Autodesk Inventor part; units mm, degrees
ref_plane "YZ Plane" through (0, 0, 0) normal (1, 0, 0) x (0, 1, 0)
ref_plane "XZ Plane" through (0, 0, 0) normal (0, 1, 0) x (-1, 0, 0)
ref_plane "XY Plane" through (0, 0, 0) normal (0, 0, 1) x (1, 0, 0)
sketch "Esquisse1" plane through (0, 0, 0) normal (0, 0, 1) x (1, 0, 0)
  line L0 (0, 0) -> (33.8, 0)
  line L1 (0, 0) -> (0, 9.5191)
  line L2 (2.3899, 12.4564) -> (30.1899, 18.2302)
  line L3 (33.8, 15.2929) -> (33.8, 0)
  arc A0 (2.3899, 12.4564) -> (0, 9.5191) centre (3, 9.5191) ccw
  arc A1 (33.8, 15.2929) -> (30.1899, 18.2302) centre (30.8, 15.2929) ccw
  point P0 (0, 11.96)
  point P1 (33.8, 18.98)
  dimension "d0" = 33.8
  dimension "d1" = 18.98
  dimension "d2" = 11.96
  dimension "d3" = 3
  dimension "d4" = 3
extrude "Extrusion1" add sketch "Esquisse1" against normal blind 2
sketch "Esquisse2" plane through (0, 0, 0) normal (0, -1, 0) x (1, 0, 0)
  line L0 (33.8, -2) -> (0, -2)
  line L1 (33.8, -2) -> (0, -2)
  line L2 (0, -2) -> (0, -11)
  line L3 (0, -11) -> (33.8, -11)
  line L4 (33.8, -11) -> (33.8, -2)
  point P0 (33.8, 0)
  dimension "d8" = 9
extrude "Extrusion2" add sketch "Esquisse2" against normal blind 2
sketch "Esquisse3" plane through (33.8, 0, -11) normal (0, 0, -1) x (-1, 0, 0)
  line L0 (0, 2) -> (33.8, 2)
  line L1 (33.8, 2) -> (33.8, 9.5191)
  line L2 (0, 15.2929) -> (0, 2)
  line L3 (0, 15.2929) -> (0, 2)
  line L4 (0, 2) -> (33.8, 2)
  line L5 (3.6101, 18.2302) -> (31.4101, 12.4564)
  arc A0 (3.6101, 18.2302) -> (0, 15.2929) centre (3, 15.2929) ccw
  arc A1 (33.8, 9.5191) -> (31.4101, 12.4564) centre (30.8, 9.5191) ccw
  point P0 (33.8, 0)
  point P1 (33.8, 11.96)
  point P2 (0, 18.98)
  dimension "d11" = 9.96
  dimension "d12" = 16.98
  dimension "d13" = 3
extrude "Extrusion3" add sketch "Esquisse3" against normal blind 2
sketch "Esquisse4" plane through (0, 0, 0) normal (0, 0, 1) x (1, 0, 0)
  line L0 (0, 0) -> (3.39, 0) construction
  line L1 (0, 0) -> (33.8, 0) construction
  line L2 (3.39, 9.1) -> (3.39, 0) construction
  circle A0 centre (3.39, 9.1) radius 2
  circle A1 centre (30.41, 9.1) radius 2
  line L3 (33.8, 0) -> (33.8, 15.2929)
  dimension "d16" = 3.39
  dimension "d17" = 9.1
  dimension "d19" = 4
  dimension "d20" = 4
  dimension "d21" = 3.39
  dimension "d26" = 9.1
extrude "Extrusion4" cut sketch "Esquisse4" against normal blind 2
sketch "Esquisse5" plane through (33.8, 0, -11) normal (0, 0, -1) x (-1, 0, 0)
  circle A0 centre (3.39, 9.1) radius 2
  circle A1 centre (3.39, 9.1) radius 2
  circle A2 centre (30.41, 9.1) radius 2
  circle A3 centre (30.41, 9.1) radius 2
  point P0 (33.8, 0)
extrude "Extrusion5" cut sketch "Esquisse5" against normal blind 2
properties part number "finger1" material "Plastique ABS"
For this review, take the finished solid that the model builds, in its own axes (mm). A direction names the side the tool comes from. Coordinates: 2 decimals unless noted, no trailing zeros. Order: outer loops, then holes, each group sorted by start corner. A loop starts at its lowest first (then second) coordinate and runs counter-clockwise, first axis right, second up. Notation, with made-up numbers: (35, 89.5) -> (61, 89.5) arc R10 cw to (61, 102.5) -> close; hole circle Ø6 at (19.25, 51.5). An arc over 180 degrees is marked (long way). Use CSV: the item, a comma, the result in double quotes. Start each with the question number.
Item 1: Draft analysis for pull direction X (two halves, no side actions). For faces 3 (the face through (33.8, 7.8, -9.2)), 4 (the face through (16.095, 15.303, -0.986)), 5 (the face through (4.465, 10.786, -0.986)), state which applies: pulls with the +X half, pulls with the -X half, needs draft (parallel to the pull), parting line crosses it, or undercut.
Item 2: Insertion check: pin 1 (5 mm diameter, centred on x = 30.41, y = 9.1, fed in from +Z); pin 2 (2 mm diameter, centred on x = 18, z = -6.5, fed in from +Y). Each pin has a flat end and moves straight along its axis. Give the tip position at first contact, or say it passes through.
Item 3: For faces 1 (the face through (17, 8, -9)), 2 (the face through (17, 7, 0)), list the 3-axis set-ups (+Z, -Z, +X, -X, +Y, -Y) from which the entire face can be reached by the end or side of a thin tool; tool diameter is ignored.
Item 4: We need section C-C, the plane x = 3.39. Give the boundary of the cut face in (y, z).
Item 5: We need section D-D, the plane x = 20. Give the boundary of the cut face in (y, z), then the cut area to 3 significant figures.
Item 6: Wall thickness on probe 1 along Z at (x, y) = (28, 11); probe 2 along Y at (x, z) = (19, -4); probe 3 along Y at (x, z) = (30.41, -10.55): over which ranges is each line inside the solid? List them lowest first.
Item 7: We need section A-A, the plane y = 3.25. Give the boundary of the cut face in (x, z).
Item 8: We need section B-B, the plane y = 9.1. Give the boundary of the cut face in (x, z), then the cut area to 3 significant figures.
Derived:
1,face 3,"pulls with the +X half"
1,face 4,"pulls with the -X half"
1,face 5,"undercut"
2,pin 1,"stops at z = 0"
2,pin 2,"stops at y = 2"
3,face 1,"+X, -X, +Y"
3,face 2,"+Z, +X, -X, +Y, -Y"
4,outline,"(0, -11) -> (7.1, -11) -> (7.1, -9) -> (2, -9) -> (2, -2) -> (7.1, -2) -> (7.1, 0) -> (0, 0) -> close; (11.1, -11) -> (12.66, -11) -> (12.66, -9) -> (11.1, -9) -> close; (11.1, -2) -> (12.66, -2) -> (12.66, 0) -> (11.1, 0) -> close"
5,outline,"(0, -11) -> (16.11, -11) -> (16.11, -9) -> (2, -9) -> (2, -2) -> (16.11, -2) -> (16.11, 0) -> (0, 0) -> close"
5,area,"78.5 mm^2"
6,probe 1,"z = -11 to -9, -2 to 0"
6,probe 2,"y = 0 to 2"
6,probe 3,"y = 0 to 7.1, 11.1 to 18.27"
7,outline,"(0, -11) -> (33.8, -11) -> (33.8, -9) -> (0, -9) -> close; (0, -2) -> (33.8, -2) -> (33.8, 0) -> (0, 0) -> close"
8,outline,"(0, -11) -> (1.39, -11) -> (1.39, -9) -> (0, -9) -> close; (0, -2) -> (1.39, -2) -> (1.39, 0) -> (0, 0) -> close; (5.39, -11) -> (28.41, -11) -> (28.41, -9) -> (5.39, -9) -> close; (5.39, -2) -> (28.41, -2) -> (28.41, 0) -> (5.39, 0) -> close; (32.41, -11) -> (33.8, -11) -> (33.8, -9) -> (32.41, -9) -> close; (32.41, -2) -> (33.8, -2) -> (33.8, 0) -> (32.41, 0) -> close"
8,area,"103 mm^2"
